Model file for the job. Use its own axes, mm. A direction names the side the tool comes from. Round coordinates to 2 decimals unless told otherwise and drop trailing zeros. Loops run counter-clockwise (first coordinate to the right, second up) from the corner with the lowest first, then second, coordinate; pieces in that order, holes last. Notation, with made-up numbers: M -3,71.25 L 12,71.25 A30 ccw 12,109.25 Z; hole C -10,-17.75 d2. An arc over 180 degrees is marked long. Use a Markdown table: item, result. Add a question column.
Item 1: Saw through at C-C on x = 1.5. Write the cut outline in (y, z).
Item 2: Tool access for faces 4 (the flat face through (13, 5, -7.5)), 5 (the flat face through (5.2, 5, 0)), 6 (the flat face through (20.2, 5, 0)): list every direction of +Z, -Z, +X, -X, +Y, -Y with a clear straight run to the whole face (end or side of a thin tool).
Item 3: Two-plate mould, pull along X, no slides. Class faces 1 (the cylindrical face through (24.636, 0.796, -10.706)), 2 (the cylindrical face through (-23.35, 0.77, -10.06)), 3 (the flat face through (0, 1, -11.43)): +X half, -X half, draft (parallel to the pull), parting line (faces both ways), or undercut.
Item 4: Pin check, flat tips, straight feed: P1, Ø4, axis at x = -13, y = 2.5, coming from the -Z side; P2, Ø1.5, axis at x = -10, z = 0, coming from the +Y side; P3, Ø1.5, axis at y = 4.5, z = 2, coming from the +X side; P4, Ø1, axis at y = 4.5, z = 7, coming from the -X side. Stop position of each tip, or through.
Item 5: Saw through at B-B on y = 4.5. Write the cut outline in (x, z), then the cut area to 3 significant figures.
Item 6: Saw through at A-A on z = 1.25. Write the cut outline in (x, y).
Item 7: Wall check: L1, parallel to X at y = 1, z = -8.89; L2, parallel to Z at x = 17.5, y = 3.25; L3, parallel to X at y = 5.25, z = 6. Give the ranges that are in metal, low to high. Write a range as from..to.
```python
from build123d import *

# Parameters (mm, degrees)
SKETCH1_W                = 50.8
SKETCH1_H                = 22.86
BOSS_EXTRUDE1_DEPTH      = 1.57
F_1_16_0_1_DOWEL_HOLE1_D = 2.54
FILLET1_R                = 2.54
SKETCH2_W                = 15
SKETCH2_H                = 15
BOSS_EXTRUDE2_DEPTH      = 6.2


with BuildPart() as part:
    # Sketch1 → Boss-Extrude1 (new body)
    with BuildSketch(Plane(origin=(0, 0, 0), x_dir=(1, 0, 0), z_dir=(0, 1, 0))):
        Rectangle(SKETCH1_W, SKETCH1_H)
    extrude(amount=BOSS_EXTRUDE1_DEPTH)

    # 1/16 (0.1) Dowel Hole1 (through all)
    with Locations(Plane(origin=(-22.86, 1.57, -8.89), x_dir=(0, 0, 1), z_dir=(0, 1, 0))):
        with Locations((0, 0), (0, 45.72), (17.78, 45.72), (17.78, 0)):
            Hole(F_1_16_0_1_DOWEL_HOLE1_D / 2)

    # Fillet1
    fillet1_edges = [part.edges().sort_by_distance(p)[0] for p in [
        (25.4, 0.785, 11.43),
        (-25.4, 0.785, 11.43),
        (-25.4, 0.785, -11.43),
        (25.4, 0.785, -11.43),
    ]]
    fillet(fillet1_edges, radius=FILLET1_R)

    # Sketch2 → Boss-Extrude2 (add)
    with BuildSketch(Plane(origin=(0, 1.57, 0), x_dir=(1, 0, 0), z_dir=(0, 1, 0))):
        with Locations((12.7, 0)):
            Rectangle(SKETCH2_W, SKETCH2_H)
    extrude(amount=BOSS_EXTRUDE2_DEPTH)


solid = part.part
```
Entries:
| question | item | result |
|---|---|---|
| 1 | outline | M 0,-11.43 L 1.57,-11.43 L 1.57,11.43 L 0,11.43 Z |
| 2 | face 4 | -Z, +X, -X, +Y |
| 2 | face 5 | +Z, -Z, -X, +Y |
| 2 | face 6 | +Z, -Z, +X, +Y |
| 3 | face 1 | +X half |
| 3 | face 2 | undercut |
| 3 | face 3 | draft |
| 4 | P1 | z = -11.43 |
| 4 | P2 | y = 1.57 |
| 4 | P3 | x = 20.2 |
| 4 | P4 | x = 5.2 |
| 5 | outline | M 5.2,-7.5 L 20.2,-7.5 L 20.2,7.5 L 5.2,7.5 Z |
| 5 | area | 225 mm2 |
| 6 | outline | M -25.4,0 L 25.4,0 L 25.4,1.57 L 20.2,1.57 L 20.2,7.77 L 5.2,7.77 L 5.2,1.57 L -25.4,1.57 Z |
| 7 | L1 | -25.4..-24.13, -21.59..21.59, 24.13..25.4 |
| 7 | L2 | -7.5..7.5 |
| 7 | L3 | 5.2..20.2 |
